Read the model definition and answer for the solid it produces. Units are mm, in the model's axes. A direction names the side the tool comes from. Coordinates: 2 decimals unless noted, no trailing zeros. Write each loop counter-clockwise with the first axis right and the second up, starting at its lowest first coordinate (ties: lowest second). Pieces come first, ordered by that corner, then holes. Notation, with made-up numbers: (56, 42.5) -> (111, 42.5) arc R22 ccw to (111, 69.5) -> close; hole circle Ø2 at (-38.75, 81). An arc over 180 degrees is marked (long way). Answer in a Markdown table with one row per item. Add a question column.
Item 1: For a pull along X with two mould halves and no side action, classify faces 4 (the face through (11.726, 1.795, -10.391)), 5 (the face through (1, -5, -19.718)), 6 (the face through (0, 7, -24.061)) as +X half, -X half, draft (parallel to the pull), parting line (faces both ways), or undercut.
Item 2: Section C-C on y = 4.25 is taken. Write down the section's boundary in (x, z).
Item 3: Straight lines are drawn through the part: line 1 (Y direction, x = 3.25, z = -28.5); line 2 (Y direction, x = -3, z = -23.25); line 3 (X direction, y = -3.75, z = -16). For each, find the intervals that lie inside material, in ascending order. Write a range as from..to.
Item 4: Which of the six approach directions +Z, -Z, +X, -X, +Y, -Y give full straight-line access (tool end or side, diameter ignored) to faces 1 (the face through (-5.809, 2.956, -21.937)), 2 (the face through (9, -0.285, -12)), 3 (the face through (4.11, 7.24, -18.45))?
Item 5: Section D-D on x = -5.75 is taken. Write down the section's boundary in (y, z).
Item 6: Given pin 1 Ø3 at (x, z) = (10, -14) entering from +Y; pin 2 Ø0.8 at (x, y) = (1.5, 7.5) entering from -Z; pin 3 Ø2 at (x, z) = (-5, -14) entering from -Y; pin 4 Ø8.5 at (y, z) = (0.14, -28.51) entering from -X, each flat-ended and moving along its own axis, determine where each tip first touches the part or whether it passes through.
Item 7: Section B-B on z = -21 is taken. Write down the section's boundary in (x, y) (3 decimals), then the cut area to 3 significant figures.
Item 8: Section A-A on y = -1 is taken. Write down the section's boundary in (x, z).
```python
from build123d import *

# Parameters (mm, degrees)
SKETCH3_R           = 8.0645
CUT_EXTRUDE1_DEPTH  = 15.24
CUT_EXTRUDE2_DEPTH  = 15.24
CUT_EXTRUDE3_DEPTH  = 12.7
BOSS_EXTRUDE1_DEPTH = 6.35
SKETCH8_R           = 1.3462
CUT_EXTRUDE4_DEPTH  = 14.605
CUT_EXTRUDE5_DEPTH  = 29.21
SKETCH10_W          = 7.112
SKETCH10_H          = 9.652
BOSS_EXTRUDE2_DEPTH = 19.05
SKETCH11_R          = 12.446
CUT_EXTRUDE6_DEPTH  = 13.97
CUT_EXTRUDE8_DEPTH  = 13.97
SKETCH14_R          = 1.3462
CUT_EXTRUDE9_DEPTH  = 13.97
CUT_EXTRUDE10_START = 21.59
CUT_EXTRUDE10_DEPTH = 21.59
BOSS_EXTRUDE3_START = 2.54
BOSS_EXTRUDE3_DEPTH = 2.54
SCALE1_SCALE        = 0.6


with BuildPart() as part:
    # Sketch1 → Revolve1 (revolve)
    with BuildSketch(Plane(origin=(0, 0, 0), x_dir=(0, 0, -1), z_dir=(1, 0, 0)), mode=Mode.PRIVATE) as revolve1_sk:
        Polygon((0, 12.446), (0, 13.335), (42.799, 13.335), (42.799, 0), (19.05, 0), (19.05, 12.446), align=None)
    revolve(revolve1_sk.sketch.rotate(Axis((0, 0, 0), (0, 0, -1)), 90), axis=Axis((0, 0, 0), (0, 0, -1)))

    # Sketch3 → Cut-Extrude1 (cut, symmetric)
    with BuildSketch(Plane(origin=(0, 0, 0), x_dir=(0, 0, -1), z_dir=(1, 0, 0))):
        with Locations((33.7058, 0)):
            Circle(SKETCH3_R)
    extrude(amount=CUT_EXTRUDE1_DEPTH, both=True, mode=Mode.SUBTRACT)

    # Sketch5 → Cut-Extrude2 (cut, symmetric)
    with BuildSketch(Plane(origin=(0, 0, 0), x_dir=(0, 0, -1), z_dir=(1, 0, 0))):
        with BuildLine():
            Line((33.7058, 9.0932), (19.939, 9.0932))
            Line((19.939, 9.0932), (19.939, 13.335))
            Line((19.939, 13.335), (43.742849638, 13.335))
            Line((43.742849638, 13.335), (43.742849638, -13.335))
            Line((43.742849638, -13.335), (19.939, -13.335))
            Line((19.939, -13.335), (19.939, -9.0932))
            Line((19.939, -9.0932), (33.7058, -9.0932))
            ThreePointArc((33.7058, -9.0932), (42.799, 0), (33.7058, 9.0932))
        make_face()
    extrude(amount=CUT_EXTRUDE2_DEPTH, both=True, mode=Mode.SUBTRACT)

    # Sketch6 → Cut-Extrude3 (cut)
    with BuildSketch(Plane.XY.offset(-19.05)):
        with BuildLine():
            Line((-6.096, 6.35), (6.096, 6.35))
            ThreePointArc((6.096, 6.35), (12.446, 0), (6.096, -6.35))
            Line((6.096, -6.35), (-6.096, -6.35))
            ThreePointArc((-6.096, -6.35), (-12.446, 0), (-6.096, 6.35))
        make_face()
    extrude(amount=-CUT_EXTRUDE3_DEPTH, mode=Mode.SUBTRACT)

    # Sketch7 → Boss-Extrude1 (add)
    with BuildSketch(Plane(origin=(0, 0, -19.939), x_dir=(-1, 0, 0), z_dir=(0, 0, -1))):
        with BuildLine():
            Line((-5.715, 9.0932), (5.715, 9.0932))
            ThreePointArc((5.715, 9.0932), (3.46993597, 10.02313597), (2.54, 12.2682))
            Line((2.54, 12.2682), (2.54, 12.832028717))
            ThreePointArc((2.54, 12.832028717), (0, 13.081), (-2.54, 12.832028717))
            Line((-2.54, 12.832028717), (-2.54, 12.2682))
            ThreePointArc((-2.54, 12.2682), (-3.46993597, 10.02313597), (-5.715, 9.0932))
        make_face()
    extrude(amount=BOSS_EXTRUDE1_DEPTH)

    # Sketch8 → Cut-Extrude4 (cut, symmetric)
    with BuildSketch(Plane(origin=(0, 0, 0), x_dir=(1, 0, 0), z_dir=(0, 1, 0))):
        with Locations(Location((0, 23.114, 0), (0, 0, 270))):
            Circle(SKETCH8_R)
    extrude(amount=CUT_EXTRUDE4_DEPTH, both=True, mode=Mode.SUBTRACT)

    # Sketch9 → Cut-Extrude5 (cut)
    with BuildSketch(Plane(origin=(0, 0, 0), x_dir=(0, 0, -1), z_dir=(1, 0, 0))):
        with BuildLine():
            Line((28.696128941, 0.7112), (13.335, 0.7112))
            ThreePointArc((13.335, 0.7112), (12.6238, 0), (13.335, -0.7112))
            Line((13.335, -0.7112), (28.696128941, -0.7112))
            Line((28.696128941, -0.7112), (28.696128941, 0.7112))
        make_face()
    extrude(amount=-CUT_EXTRUDE5_DEPTH, mode=Mode.SUBTRACT)

    # Sketch10 → Boss-Extrude2 (add)
    with BuildSketch(Plane(origin=(0, 0, 0), x_dir=(0, 0, -1), z_dir=(1, 0, 0))):
        with Locations((3.556, 0)):
            Rectangle(SKETCH10_W, SKETCH10_H)
    extrude(amount=BOSS_EXTRUDE2_DEPTH)

    # Sketch11 → Cut-Extrude6 (cut)
    with BuildSketch(Plane.XY):
        Circle(SKETCH11_R)
    extrude(amount=-CUT_EXTRUDE6_DEPTH, mode=Mode.SUBTRACT)

    # Sketch13 → Cut-Extrude8 (cut)
    with BuildSketch(Plane.XY):
        with BuildLine():
            Line((19.689857662, 4.826), (19.689857662, -4.826))
            Line((19.689857662, -4.826), (18.428570862, -4.826))
            ThreePointArc((18.428570862, -4.826), (19.05, 0), (18.428570862, 4.826))
            Line((18.428570862, 4.826), (19.689857662, 4.826))
        make_face()
    extrude(amount=-CUT_EXTRUDE8_DEPTH, mode=Mode.SUBTRACT)

    # Sketch14 → Cut-Extrude9 (cut)
    with BuildSketch(Plane(origin=(0, 4.826, 0), x_dir=(1, 0, 0), z_dir=(0, 1, 0))):
        with Locations(Location((15.429829434, 3.556, 0), (0, 0, 270))):
            Circle(SKETCH14_R)
    extrude(amount=-CUT_EXTRUDE9_DEPTH, mode=Mode.SUBTRACT)

    # Sketch15 → Cut-Extrude10 (cut)
    with BuildSketch(Plane(origin=(0, 0, 0), x_dir=(0, 0, -1), z_dir=(1, 0, 0)).offset(CUT_EXTRUDE10_START)):
        with BuildLine():
            Line((0, 0.7112), (25.672721212, 0.7112))
            ThreePointArc((25.672721212, 0.7112), (25.6413, 0), (25.672721212, -0.7112))
            Line((25.672721212, -0.7112), (0, -0.7112))
            Line((0, -0.7112), (0, 0.7112))
        make_face()
    extrude(amount=-CUT_EXTRUDE10_DEPTH, mode=Mode.SUBTRACT)

    # Sketch16 → Boss-Extrude3 (add)
    with BuildSketch(Plane.XY.offset(-19.05).offset(BOSS_EXTRUDE3_START)):
        with BuildLine():
            Line((-0.5715, 10.641698231), (-0.5715, 10.367746169))
            Line((-0.5715, 10.367746169), (0.5715, 10.367746169))
            Line((0.5715, 10.367746169), (0.5715, 10.641698231))
            ThreePointArc((0.5715, 10.641698231), (1.154243176, 11.870771042), (2.474643275, 12.197502066))
            ThreePointArc((2.474643275, 12.197502066), (0, 12.446), (-2.474643275, 12.197502066))
            ThreePointArc((-2.474643275, 12.197502066), (-1.154243176, 11.870771042), (-0.5715, 10.641698231))
        make_face()
    extrude(amount=-BOSS_EXTRUDE3_DEPTH)


with BuildPart() as part_1:
    # Scale1: scaled about (1.039780089, 0.353442255, -20.719141089)
    add(part.part.scale(SCALE1_SCALE).moved(Location((0.415912036, 0.141376902, -8.287656436))))


solid = part_1.part
```
Results below:
| question | item | result |
|---|---|---|
| 1 | face 4 | +X half |
| 1 | face 5 | undercut |
| 1 | face 6 | draft |
| 2 | outline | (-6.45, -32.1) -> (7.28, -32.1) -> (7.28, -31.07) -> (-6.45, -31.07) -> close; (-6.45, -25.96) -> (7.28, -25.96) -> (7.28, -8.29) -> (6.65, -8.29) -> (6.65, -19.72) -> (-5.82, -19.72) -> (-5.82, -8.29) -> (-6.45, -8.29) -> close; hole circle Ø1.62 at (0.42, -22.16) |
| 3 | line 1 | y = -5.31..-4.7, 4.98..5.6 |
| 3 | line 2 | y = -5.31..-3.67, 3.95..5.6 |
| 3 | line 3 | x = -6.58..-5.96, 6.79..7.41 |
| 4 | face 1 | +Z |
| 4 | face 2 | +Z, +X |
| 4 | face 3 | -Z |
| 5 | outline | (-4.96, -30.45) arc R5.46 ccw to (5.24, -30.45) -> (5.24, -8.29) -> (4.35, -8.29) -> (4.35, -19.72) -> (3.01, -19.72) -> (3.01, -24.61) arc R4.84 cw (long way) to (-2.73, -24.61) -> (-2.73, -19.72) -> (-4.07, -19.72) -> (-4.07, -8.29) -> (-4.96, -8.29) -> close |
| 6 | pin 1 | stops at y = 3.04 |
| 6 | pin 2 | stops at z = -24.06 |
| 6 | pin 3 | stops at y = -6.53 |
| 6 | pin 4 | passes through |
| 7 | outline | (-7.574, -0.285) arc R8.001 ccw to (-5.436, -5.315) -> (6.268, -5.315) arc R8.001 ccw to (8.406, -0.285) -> (7.86, -0.285) arc R3.81 cw to (4.074, -3.669) -> (-3.242, -3.669) arc R3.81 cw to (-7.028, -0.285) -> close; (-7.574, 0.568) -> (-7.028, 0.568) arc R3.81 cw to (-3.242, 3.951) -> (4.074, 3.951) arc R3.81 cw to (7.86, 0.568) -> (8.406, 0.568) arc R8.001 ccw to (6.268, 5.597) -> (3.845, 5.597) arc R1.905 cw to (1.94, 7.502) -> (1.94, 7.841) arc R7.849 ccw to (-1.108, 7.841) -> (-1.108, 7.502) arc R1.905 cw to (-3.013, 5.597) -> (-5.436, 5.597) arc R8.001 ccw to start |
| 7 | area | 66.4 mm2 |
| 8 | outline | (-7.5, -33.85) -> (8.34, -33.85) -> (8.34, -33.21) -> (-7.5, -33.21) -> close; (-7.5, -23.81) -> (-6.88, -23.81) -> (-6.88, -19.72) -> (-6.96, -19.72) -> (-6.96, -8.29) -> (-7.5, -8.29) -> close; (7.71, -23.81) -> (8.34, -23.81) -> (8.34, -12.55) -> (11.79, -12.55) -> (11.79, -8.29) -> (7.8, -8.29) -> (7.8, -19.72) -> (7.71, -19.72) -> close; hole circle Ø1.62 at (9.67, -10.42) |
